Design review of the part built by this model. Coordinates are the model's own, in mm. A direction names the side the tool comes from. Coordinates: 2 decimals unless noted, no trailing zeros. Write each loop counter-clockwise with the first axis right and the second up, starting at its lowest first coordinate (ties: lowest second). Pieces come first, ordered by that corner, then holes. Notation, with made-up numbers: (-12.75, -26) -> (31.25, -26) arc R17 ccw to (31.25, -1) -> close; hole circle Ø5 at (-5, 80.5). An arc over 180 degrees is marked (long way). Answer in a Markdown table with one row per item. Add a question column.
Item 1: Take a section at A-A, the plane x = 5.4. Write out the cut boundary in (y, z).
Item 2: Take a section at B-B, the plane y = 3.5. Write out the cut boundary in (x, z), and give its area (3 significant figures).
Item 3: To check wall thickness, follow line 1 (Y direction, x = 5.75, z = -1.5). State the ranges of the line that lie inside material, in increasing order.
Item 4: Draft analysis for pull direction Y (two halves, no side actions). For faces 1 (the face through (5, -5, 47)), 2 (the face through (5, 0, 0)), 3 (the face through (5, -52.5, 46)), 4 (the face through (6, -1, 21)), state which applies: released by +Y, released by -Y, zero draft, split by the parting line, or undercut.
Item 5: For faces 5 (the face through (5, 0, 45)), 6 (the face through (5, -55, 0)), 7 (the face through (5, 55, 0)), 8 (the face through (5, 55, 45)), 9 (the face through (5, 5, -3)), list the 3-axis set-ups (+Z, -Z, +X, -X, +Y, -Y) from which the entire face can be reached by the end or side of a thin tool; tool diameter is ignored.
Item 6: Clearance check with flat-ended pins moving along their axes: P1, Ø0.6, axis at x = 5, z = 46.5, coming from the -Y side; P2, Ø1, axis at x = 5.5, y = 54.5, coming from the -Z side. State where each tip first meets the part, or that it passes through.
from build123d import *

# Parameters (mm, degrees)
ESTRUSIONE_ESTRUSIONE1_DEPTH      = 48
ESTRUSIONE_ESTRUSIONE1_DEPTH_BACK = 6
SCHIZZO1_W                        = 2
SCHIZZO1_H                        = 105
TAGLIO_ESTRUSIONE1_DEPTH          = 10
SCHIZZO3_W                        = 2
SCHIZZO3_H                        = 45
ESTRUSIONE_ESTRUSIONE2_DEPTH      = 5


with BuildPart() as part:
    # Schizzo1 → Estrusione-Estrusione1 (new, two sides: drawn at the far end of the back side and taken through both)
    with BuildSketch(Plane.XY.offset(-ESTRUSIONE_ESTRUSIONE1_DEPTH_BACK)):
        with Locations((5, 0)):
            Rectangle(SCHIZZO1_W, SCHIZZO1_H)
    extrude(amount=ESTRUSIONE_ESTRUSIONE1_DEPTH + ESTRUSIONE_ESTRUSIONE1_DEPTH_BACK)

    # Schizzo2 → Taglio-Estrusione1 (cut)
    with BuildSketch(Plane(origin=(6, 0, 0), x_dir=(0, 0, -1), z_dir=(1, 0, 0))):
        Polygon((-48, -5), (-45, -5), (-45, 0), (-45, 5), (-48, 5), align=None)
        Polygon((6, -5), (0, -5), (0, 0), (0, 5), (6, 5), align=None)
    extrude(amount=-TAGLIO_ESTRUSIONE1_DEPTH, mode=Mode.SUBTRACT)

    # Schizzo3 → Estrusione-Estrusione2 (add)
    with BuildSketch(Plane.XZ.offset(52.5)):
        with Locations((5, 22.5)):
            Rectangle(SCHIZZO3_W, SCHIZZO3_H)
    estrusione_estrusione2 = extrude(amount=ESTRUSIONE_ESTRUSIONE2_DEPTH)

    # Specchia1: Estrusione-Estrusione2 across plane
    add(estrusione_estrusione2.mirror(Plane(origin=(0, 0, 0), x_dir=(0, 0, 1), z_dir=(0, -1, 0))))


solid = part.part
Answers:
| question | item | result |
|---|---|---|
| 1 | outline | (-57.5, 0) -> (-52.5, 0) -> (-52.5, -6) -> (-5, -6) -> (-5, 0) -> (5, 0) -> (5, -6) -> (52.5, -6) -> (52.5, 0) -> (57.5, 0) -> (57.5, 45) -> (52.5, 45) -> (52.5, 48) -> (5, 48) -> (5, 45) -> (-5, 45) -> (-5, 48) -> (-52.5, 48) -> (-52.5, 45) -> (-57.5, 45) -> close |
| 2 | outline | (4, 0) -> (6, 0) -> (6, 45) -> (4, 45) -> close |
| 2 | area | 90.0 mm^2 |
| 3 | line 1 | y = -52.5 to -5, 5 to 52.5 |
| 4 | face 1 | undercut |
| 4 | face 2 | undercut |
| 4 | face 3 | released by -Y |
| 4 | face 4 | zero draft |
| 5 | face 5 | +Z, +X, -X |
| 5 | face 6 | -Z, +X, -X, -Y |
| 5 | face 7 | -Z, +X, -X, +Y |
| 5 | face 8 | +Z, +X, -X, +Y |
| 5 | face 9 | -Z, +X, -X |
| 6 | P1 | stops at y = -52.5 |
| 6 | P2 | stops at z = 0 |
